Part print with two shaded views. Sizes in mm from the minimum x, y, z corner. Round coordinates to 2 decimals unless told otherwise and drop trailing zeros. Loops run counter-clockwise (first coordinate to the right, second up) from the corner with the lowest first, then second, coordinate; pieces in that order, holes last. Notation, with made-up numbers: (23, 45.5) -> (39, 45.5) arc R18 ccw to (39, 67.5) -> close; hole circle Ø2 at (9.5, -36.75). An arc over 180 degrees is marked (long way). Put each result on its own line as item: value. Start each with the question number.
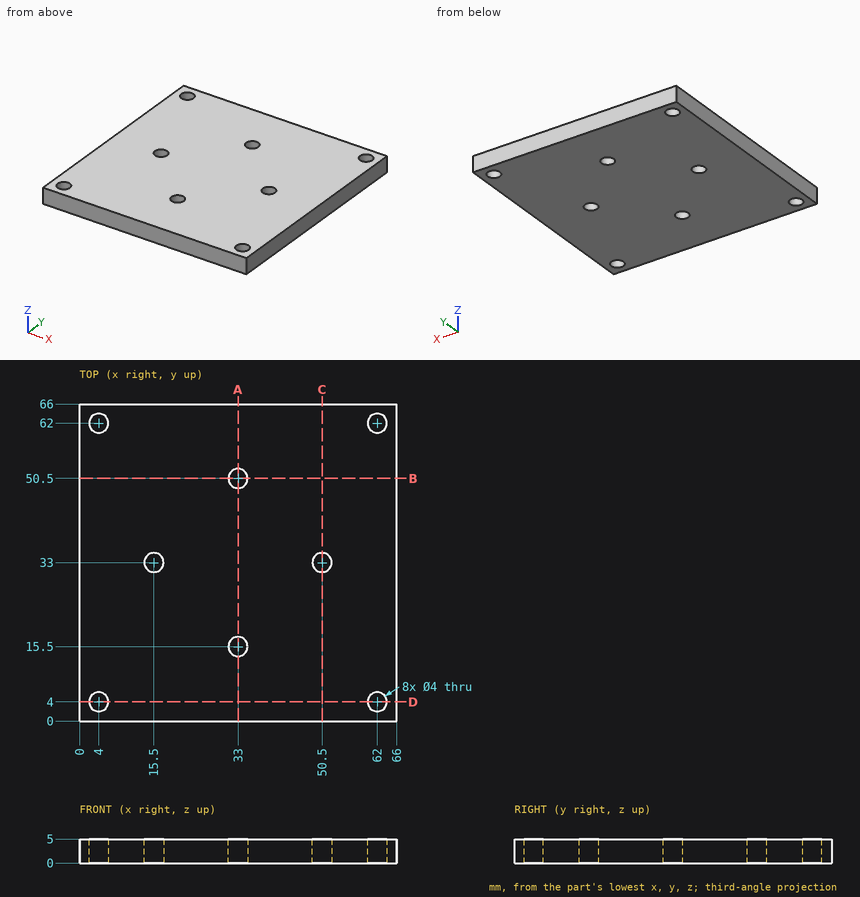
Item 1: Drop a flat-ended pin along its axis: pin 1 (3.5 mm diameter, centred on x = 62, y = 62, fed in from +Z). Give the stop position or say it passes through.
Item 2: Cut at A-A on x = 33. Write the cut outline in (y, z), then the cut area to 3 significant figures.
Item 3: Cut at D-D on y = 4. Write the cut outline in (x, z).
Item 4: Cut at B-B on y = 50.5. Write the cut outline in (x, z), then the cut area to 3 significant figures.
Item 5: Wall check: line 1 (Y direction, x = 33, z = 2.1); line 2 (Y direction, x = 4, z = 1.25); line 3 (X direction, y = 49, z = 3.8). Give the ranges that are in metal, low to high. Write a range as from..to.
Ans:
1. pin 1: passes through
2. outline: (0, 0) -> (13.5, 0) -> (13.5, 5) -> (0, 5) -> close; (17.5, 0) -> (48.5, 0) -> (48.5, 5) -> (17.5, 5) -> close; (52.5, 0) -> (66, 0) -> (66, 5) -> (52.5, 5) -> close
2. area: 290 mm2
3. outline: (0, 0) -> (2, 0) -> (2, 5) -> (0, 5) -> close; (6, 0) -> (60, 0) -> (60, 5) -> (6, 5) -> close; (64, 0) -> (66, 0) -> (66, 5) -> (64, 5) -> close
4. outline: (0, 0) -> (31, 0) -> (31, 5) -> (0, 5) -> close; (35, 0) -> (66, 0) -> (66, 5) -> (35, 5) -> close
4. area: 310 mm2
5. line 1: y = 0..13.5, 17.5..48.5, 52.5..66
5. line 2: y = 0..2, 6..60, 64..66
5. line 3: x = 0..31.68, 34.32..66
